Part print with two shaded views. Sizes in mm from the minimum x, y, z corner. A direction names the side the tool comes from. Give positions to 0.01 mm unless a question says otherwise; leave off trailing zeros. Order: outer loops, then holes, each group sorted by start corner. A loop starts at its lowest first (then second) coordinate and runs counter-clockwise, first axis right, second up. Notation, with made-up numbers: (3, -33.5) -> (54, -33.5) arc R12 cw to (54, -15.5) -> close; hole circle Ø8 at (15.5, 6.25). An arc over 180 degrees is marked (long way). Write item = value, one per line. Start each with the question number.
Item 1: Drill centre lines: line 1 along X through (y, z) = (18, 9.5); line 2 along X through (y, z) = (14, 22.75); line 3 along Y through (x, z) = (7.5, 19). Where is each one in solid material? Low to high.
Item 2: Band-saw the part on D-D on x = 19. Write the cut outline in (y, z), plus the area to 3 significant figures.
Item 3: Band-saw the part on A-A on y = 14.5. Write the cut outline in (x, z).
Item 4: Tool access for the marked faces 1 and 2: list every direction of +Z, -Z, +X, -X, +Y, -Y with a clear straight run to the whole face (end or side of a thin tool).
Item 5: Band-saw the part on B-B on y = 22.25. Write the cut outline in (x, z), plus the area to 3 significant figures.
Item 6: Band-saw the part on C-C on z = 15.75. Write the cut outline in (x, y).
Item 7: Flat gauge pin, fed straight in: P1, Ø1, axis at x = 13, z = 10, coming from the +Y side. Where does the tip first touch, or does it go through?
Item 8: Pull direction X, two halves, no side cores. Call the marked faces 3, 4, 5 and 6: +X half, -X half, draft (parallel to the pull), parting line (faces both ways), or undercut.
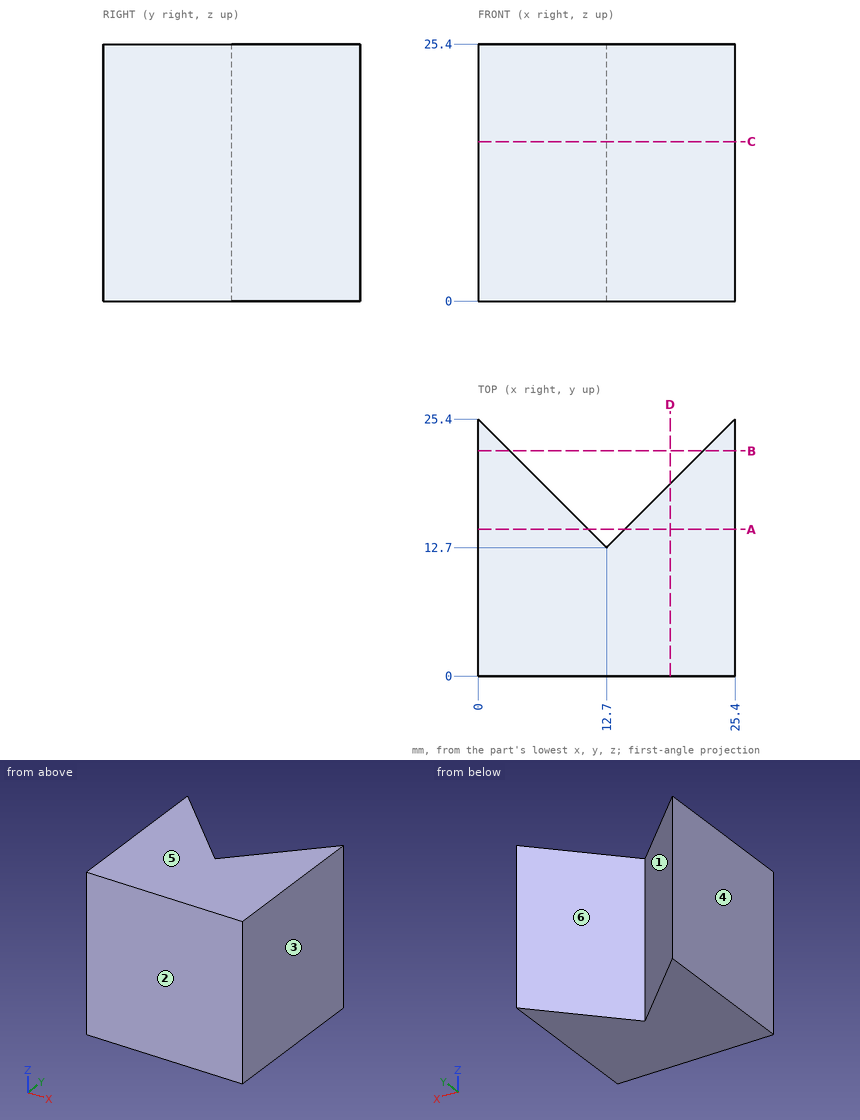
Values found:
q1.line_1 = 0 to 7.4, 18 to 25.4
q1.line_2 = 0 to 11.4, 14 to 25.4
q1.line_3 = 0 to 17.9
q2.outline = (0, 0) -> (19, 0) -> (19, 25.4) -> (0, 25.4) -> close
q2.area = 483 mm^2
q3.outline = (0, 0) -> (10.9, 0) -> (10.9, 25.4) -> (0, 25.4) -> close; (14.5, 0) -> (25.4, 0) -> (25.4, 25.4) -> (14.5, 25.4) -> close
q4.face_1 = +Z, -Z, +Y
q4.face_2 = +Z, -Z, +X, -X, -Y
q5.outline = (0, 0) -> (3.15, 0) -> (3.15, 25.4) -> (0, 25.4) -> close; (22.25, 0) -> (25.4, 0) -> (25.4, 25.4) -> (22.25, 25.4) -> close
q5.area = 160 mm^2
q6.outline = (0, 0) -> (25.4, 0) -> (25.4, 25.4) -> (12.7, 12.7) -> (0, 25.4) -> close
q7.P1 = 13.5
q8.face_3 = +X half
q8.face_4 = -X half
q8.face_5 = draft
q8.face_6 = undercut
